from build123d import *

# Parameters (mm, degrees)
F0_R            = 15.961960717
F0_R_2          = 3.96875
F0_R_3          = 3.175
F0_R_4          = 1.7272
F1_DEPTH        = 3.175
F3_DEPTH        = 3.175
F3_COPIES_COUNT = 12


# Not quite as in the source:
# - a pattern or mirror of a feature is missing from the dataset's text; its kind, count and spacing are read off the source's solid


with BuildPart() as f1:
    # F0 (on Top) → F1 (new body)
    with BuildSketch(Plane.XY):
        Circle(F0_R)
        with Locations((-6.1739260832, -6.1739260832)):
            Circle(F0_R_2, mode=Mode.SUBTRACT)
        Circle(F0_R_3, mode=Mode.SUBTRACT)
        with Locations((6.1739260832, -6.1739260832)):
            Circle(F0_R_4, mode=Mode.SUBTRACT)
        with Locations((-6.1739260832, 6.1739260832)):
            Circle(F0_R_4, mode=Mode.SUBTRACT)
        with Locations((6.1739260832, 6.1739260832)):
            Circle(F0_R_2, mode=Mode.SUBTRACT)
    extrude(amount=F1_DEPTH)

    # F2 (on face) → F3 (cut, through all)
    with BuildSketch(Plane.XY.offset(3.175)):
        with BuildLine():
            Line((-1.0271880853, 3.8335181231), (-0.8217504682, 3.0668144985))
            ThreePointArc((-0.8217504682, 3.0668144985), (-0.4144206603, 3.1478374349), (0, 3.175))
            Line((0, 3.175), (0, 3.96875))
            ThreePointArc((0, 3.96875), (-0.5180258254, 3.9347967936), (-1.0271880853, 3.8335181231))
        make_face()
    f3 = extrude(amount=-F3_DEPTH, mode=Mode.SUBTRACT)

    # F3_copies: F3 ×12 about axis
    f3_copies_axis = Axis((0, 0, 0), (0, 0, 1))
    for i in range(1, F3_COPIES_COUNT):
        add(f3.rotate(f3_copies_axis, i * 360 / F3_COPIES_COUNT), mode=Mode.SUBTRACT)


solid = f1.part
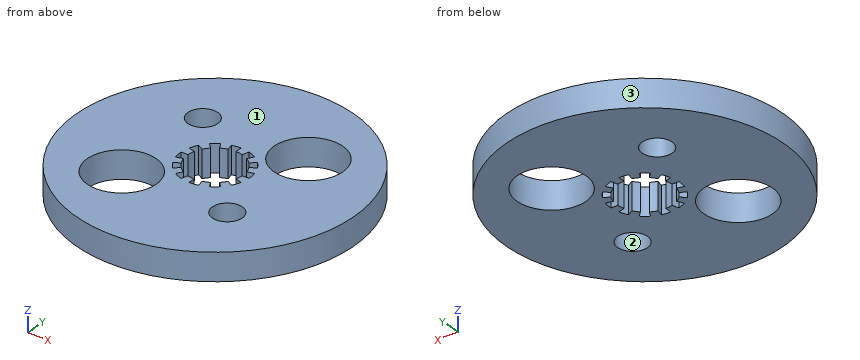
Read the model definition and answer for the solid it produces. Units are mm, in the model's axes. Face numbers are marked on the shaded views. Coordinates: 2 decimals unless noted, no trailing zeros. Loops run counter-clockwise (first coordinate to the right, second up) from the corner with the lowest first, then second, coordinate; pieces in that order, holes last. Notation, with made-up numbers: (14.25, -4.75) -> (72.25, -4.75) arc R6 cw to (72.25, 5.25) -> close; hole circle Ø2 at (62.5, -19.5). An arc over 180 degrees is marked (long way). Write item = value, one per line. Start each with the question number.
1) The part is cut by section A-A, the plane x = -7.5. Determine the outline of the cut face in (y, z) (3 decimals).
2) Find the intervals of material crossed by L1, parallel to X at y = 6.5, z = 3.05; L2, parallel to X at y = -7, z = 1.25; L3, parallel to Y at x = -5, z = 2.75, in increasing order. Write a range as from..to.
3) Given P1, Ø6, axis at x = -2.5, y = -7.5, coming from the +Z side (3 decimals); P2, Ø0.9, axis at x = 3.5, z = 2, coming from the +Y side; P3, Ø0.9, axis at y = -3.5, z = 1.5, coming from the +X side; P4, Ø0.9, axis at y = 3.5, z = 1.5, coming from the -X side, each flat-ended and moving along its own axis, determine where each tip first touches the part or whether it passes through.
4) The part is cut by section D-D, the plane x = 12. Determine the outline of the cut face in (y, z) (3 decimals).
5) The mould has two halves that part along X. Classify the marked faces 1, 2 and 3: pulls with the +X half, pulls with the -X half, needs draft (parallel to the pull), parting line crosses it, or undercut.
6) The part is cut by section C-C, the plane z = 1.5. State how many separate pieces and enclosed holes the cut face has, plus the area to 3 significant figures.
7) The part is cut by section B-B, the plane y = 7.5. Determine the outline of the cut face in (x, z) (3 decimals).
Result:
q1.outline = (-14.09, 0) -> (-9.915, 0) -> (-9.915, 3.175) -> (-14.09, 3.175) -> close; (-2.433, 0) -> (5.067, 0) -> (5.067, 3.175) -> (-2.433, 3.175) -> close; (7.281, 0) -> (14.09, 0) -> (14.09, 3.175) -> (7.281, 3.175) -> close
q2.L1 = -14.58..-7.87, -4.48..2.22, 10.13..14.58
q2.L2 = -14.35..-10.06, -2.29..4.66, 7.69..14.35
q2.L3 = -15.16..-9.97, -2.38..4.91, 7.44..15.16
q3.P1 = 3.175
q3.P2 = 15.67
q3.P3 = 15.67
q3.P4 = -15.67
q4.outline = (-10.525, 0) -> (10.525, 0) -> (10.525, 3.175) -> (-10.525, 3.175) -> close
q5.face_1 = needs draft
q5.face_2 = undercut
q5.face_3 = parting line crosses it
q6.separate_pieces = 1
q6.enclosed_holes = 5
q6.area = 642 mm²
q7.outline = (-14.09, 0) -> (-7.281, 0) -> (-7.281, 3.175) -> (-14.09, 3.175) -> close; (-5.067, 0) -> (2.433, 0) -> (2.433, 3.175) -> (-5.067, 3.175) -> close; (9.915, 0) -> (14.09, 0) -> (14.09, 3.175) -> (9.915, 3.175) -> close
